```python
from build123d import *

# Parameters (mm, degrees)
F0_R        = 2.2225
F0_R_2      = 2.54
F0_R_3      = 1.5875
F0_W        = 79.375
F0_H        = 6.35
F1_DEPTH    = 0.9525
F2_T1_DEPTH = 1.905
F3_W        = 3.4798
F3_H        = 1.7145
F3_W_2      = 1.7272
F3_H_2      = 15.24
F3_W_3      = 91.7488066308
F3_H_3      = 1.7272
F3_W_4      = 2.9169933692
F4_DEPTH    = 3.175


# Not quite as in the source:
# - a fillet or chamfer that OpenCascade refuses, or shapes differently, is made with other operations: its cross-section is extruded or revolved along the edge and cut away or added
# - a feature names something its author has since deleted; it is built from what else it names


with BuildPart() as f1:
    # F0 (on Front) → F1 (new body, symmetric)
    with BuildSketch(Plane.XZ):
        Polygon((-50.8, 27.94), (-50.8, 0), (-44.45, 0), (-44.45, 6.35), (-44.45, 17.145), (34.925, 14.3731639216), (34.925, 6.35), (34.925, 0), (50.8, 0), (50.8, 27.94), align=None)
        with Locations((42.8625, 11.7475)):
            Circle(F0_R, mode=Mode.SUBTRACT)
        Polygon((-44.45, 21.59), (28.3304192035, 21.59), (28.3304192035, 17.145), (-44.45, 19.6865482425), align=None, mode=Mode.SUBTRACT)
        with Locations((33.655, 18.415)):
            Circle(F0_R_2, mode=Mode.SUBTRACT)
        with Locations((42.8625, 18.415)):
            Circle(F0_R_3, mode=Mode.SUBTRACT)
        with Locations((-4.7625, 3.175)):
            Rectangle(F0_W, F0_H)
    extrude(amount=F1_DEPTH, both=True)

    # F2: fillet of radius 5.08 on 4 edges, made by hand

    # F2_s2 → F2_t1 (join)
    with BuildSketch(Plane.XZ.offset(-0.9525)):
        with BuildLine():
            ThreePointArc((-39.1927105568, 16.9614114072), (-42.8988645219, 15.5387521917), (-44.45, 11.8845060059))
            Line((-44.45, 11.8845060059), (-44.45, 17.145))
            Line((-44.45, 17.145), (-39.1927105568, 16.9614114072))
        make_face()
        with BuildLine():
            ThreePointArc((34.925, 9.4674649456), (33.4992461857, 12.9963294675), (30.0222894432, 14.5443703468))
            Line((30.0222894432, 14.5443703468), (34.925, 14.3731639216))
            Line((34.925, 14.3731639216), (34.925, 9.4674649456))
        make_face()
        with BuildLine():
            ThreePointArc((-44.45, 21.59), (-42.7347440797, 20.1271540197), (-40.5553991831, 19.5505457851))
            Line((-40.5553991831, 19.5505457851), (-44.45, 19.6865482425))
            Line((-44.45, 19.6865482425), (-44.45, 21.59))
        make_face()
        with BuildLine():
            ThreePointArc((28.3304192035, 21.59), (26.5399663684, 18.4773950775), (23.1386411982, 17.326300883))
            Line((23.1386411982, 17.326300883), (28.3304192035, 17.145))
            Line((28.3304192035, 17.145), (28.3304192035, 21.59))
        make_face()
    extrude(amount=F2_T1_DEPTH)

    # F3 (on Front) → F4 (join)
    with BuildSketch(Plane.XZ):
        with Locations((-49.0601, 5.49275)):
            Rectangle(F3_W, F3_H)
        with Locations((-46.4566, 13.97)):
            Rectangle(F3_W_2, F3_H_2)
        with Locations((-46.4566, 5.49275)):
            Rectangle(F3_W_2, F3_H)
        with Locations((0.2814033154, 5.49275)):
            Rectangle(F3_W_3, F3_H)
        with Locations((-46.4566, 22.4536)):
            Rectangle(F3_W_2, F3_H_3)
        with Locations((-49.0601, 22.4536)):
            Rectangle(F3_W, F3_H_3)
        with Locations((47.0194066308, 13.97)):
            Rectangle(F3_W_2, F3_H_2)
        with Locations((47.0194066308, 5.49275)):
            Rectangle(F3_W_2, F3_H)
        with Locations((0.2814033154, 22.4536)):
            Rectangle(F3_W_3, F3_H_3)
        with Locations((49.3415033154, 5.49275)):
            Rectangle(F3_W_4, F3_H)
        with Locations((47.0194066308, 22.4536)):
            Rectangle(F3_W_2, F3_H_3)
        with Locations((49.3415033154, 22.4536)):
            Rectangle(F3_W_4, F3_H_3)
    extrude(amount=F4_DEPTH)


solid = f1.part
```
Build history of the part. All positions in model axes, mm. A direction names the side the tool comes from. Give positions to 0.01 mm unless a question says otherwise; leave off trailing zeros. Loops run counter-clockwise (first coordinate to the right, second up) from the corner with the lowest first, then second, coordinate; pieces in that order, holes last. Notation, with made-up numbers: (87.5, 88.5) - (118.5, 88.5) arc R31 ccw to (118.5, 115.5) - close; hole circle Ø4 at (67.25, 67). An arc over 180 degrees is marked (long way). Use a Markdown table: item, result.
(1) Drop flat-ended pins along their axis: pin 1 Ø1.8 at (y, z) = (-2.5, 10.5) entering from -X; pin 2 Ø1.1 at (x, y) = (22, -2) entering from +Z; pin 3 Ø3 at (x, z) = (42.86, 18.42) entering from +Y; pin 4 Ø0.9 at (x, z) = (49, 14.5) entering from -Y. Give the stop position or say it passes through.
Taken from the geometry:
| item | result |
|---|---|
| pin 1 | x = -47.32 |
| pin 2 | z = 23.32 |
| pin 3 | through |
| pin 4 | y = -0.95 |
(2) Which spindle directions (+Z, -Z, +X, -X, +Y, -Y) get a long thin tool onto all of the face, cutting with end or side? Do faces 5 (the face through (1, -2, 23.317)), 6 (the face through (49, -0.952, 14)), 7 (the face through (-49, -0.952, 14)), 8 (the face through (0, -1, 21.59)), 9 (the face through (34.925, 0, 8)). Say none if no direction does.
Taken from the geometry:
| item | result |
|---|---|
| face 5 | +Z, +X, -X, -Y |
| face 6 | +X, -Y |
| face 7 | -X, -Y |
| face 8 | -Y |
| face 9 | +Y, -Y |
(3) Band-saw the part on A-A (y = -2.4). Give the cut face in (x, z), and give its area (3 significant figures).
Taken from the geometry:
| item | result |
|---|---|
| outline | (-50.8, 4.64) - (50.8, 4.64) - (50.8, 6.35) - (47.88, 6.35) - (47.88, 21.59) - (50.8, 21.59) - (50.8, 23.32) - (-50.8, 23.32) - (-50.8, 21.59) - (-47.32, 21.59) - (-47.32, 6.35) - (-50.8, 6.35) - close; hole (-45.59, 6.35) - (46.16, 6.35) - (46.16, 21.59) - (-45.59, 21.59) - close |
| area | 402 mm2 |
(4) Pull direction X, two halves, no side cores. Call faces 1 (the face through (50.8, 0, 14)), 2 (the face through (-47.32, -2, 14)), 3 (the face through (0, -3.175, 22)), 4 (the face through (14, -0.952, 16)): +X half, -X half, draft (parallel to the pull), parting line (faces both ways), or undercut.
Taken from the geometry:
| item | result |
|---|---|
| face 1 | +X half |
| face 2 | -X half |
| face 3 | draft |
| face 4 | undercut |
(5) Wall check: line 1 along X through (y, z) = (-2.8, 16.5); line 2 along Z through (x, y) = (39, -1.85). Give the ranges that are in metal, low to high.
Taken from the geometry:
| item | result |
|---|---|
| line 1 | -47.32 to -45.59, 46.16 to 47.88 |
| line 2 | 4.64 to 6.35, 21.59 to 23.32 |
(6) Band-saw the part on B-B (x = -13). Give the number of separate pieces and of enclosed holes in the cut face, and give its area (3 significant figures).
Taken from the geometry:
| item | result |
|---|---|
| separate pieces | 3 |
| enclosed holes | 0 |
| area | 36.7 mm2 |
